```python
from build123d import *

# Parameters (mm, degrees)
SKETCH2_W                 = 80
SKETCH2_H                 = 211
SKETCH2_W_2               = 53.6
SKETCH2_H_2               = 11.7
BOSS_EXTRUDE1_DEPTH       = 2
M3X0_5_TAPPED_HOLE1_D     = 2.5
M3X0_5_TAPPED_HOLE1_DEPTH = 10
M3X0_5_TAPPED_HOLE1_TIP   = 0.751075774
SKETCH7_R                 = 3
CUT_EXTRUDE1_DEPTH        = 2


with BuildPart() as part:
    # Sketch2 → Boss-Extrude1 (new body)
    with BuildSketch(Plane.XY):
        with Locations((40, 105.5)):
            Rectangle(SKETCH2_W, SKETCH2_H)
        with Locations((40, 161.75)):
            Rectangle(SKETCH2_W_2, SKETCH2_H_2, mode=Mode.SUBTRACT)
    extrude(amount=BOSS_EXTRUDE1_DEPTH)

    # M3x0.5 Tapped Hole1
    with Locations(Plane(origin=(0, 0, 0), x_dir=(-1, 0, 0), z_dir=(0, 0, -1))):
        with Locations((-75, 196), (-5, 196), (-75, 23), (-5, 23)):
            Hole(M3X0_5_TAPPED_HOLE1_D / 2, depth=M3X0_5_TAPPED_HOLE1_DEPTH)
            with Locations((0, 0, -(M3X0_5_TAPPED_HOLE1_DEPTH + M3X0_5_TAPPED_HOLE1_TIP / 2))):  # 118° drill point
                Cone(0, M3X0_5_TAPPED_HOLE1_D / 2, M3X0_5_TAPPED_HOLE1_TIP, mode=Mode.SUBTRACT)

    # Sketch7 → Cut-Extrude1 (cut)
    with BuildSketch(Plane(origin=(0, 0, 0), x_dir=(-1, 0, 0), z_dir=(0, 0, -1))):
        with Locations((-75, 186)):
            Circle(SKETCH7_R)
        with Locations((-75, 139.2)):
            Circle(SKETCH7_R)
        with Locations((-75, 109.2)):
            Circle(SKETCH7_R)
        with Locations((-75, 79.2)):
            Circle(SKETCH7_R)
        with Locations((-75, 50.2)):
            Circle(SKETCH7_R)
        with Locations((-75, 30.2)):
            Circle(SKETCH7_R)
        with Locations((-5, 186)):
            Circle(SKETCH7_R)
        with Locations((-5, 139.2)):
            Circle(SKETCH7_R)
        with Locations((-5, 109.2)):
            Circle(SKETCH7_R)
        with Locations((-5, 79.2)):
            Circle(SKETCH7_R)
        with Locations((-5, 50.2)):
            Circle(SKETCH7_R)
        with Locations((-5, 30.2)):
            Circle(SKETCH7_R)
        with Locations((-70.3, 13)):
            Circle(SKETCH7_R)
        with Locations((-60, 205)):
            Circle(SKETCH7_R)
        with Locations((-20, 205)):
            Circle(SKETCH7_R)
        with Locations((-60, 6)):
            Circle(SKETCH7_R)
        with Locations((-20, 6)):
            Circle(SKETCH7_R)
        with Locations((-9.7, 13)):
            Circle(SKETCH7_R)
    extrude(amount=-CUT_EXTRUDE1_DEPTH, mode=Mode.SUBTRACT)


solid = part.part
```
The model under review builds one solid part; all positions refer to its coordinate system, in mm. Give positions to 0.01 mm unless a question says otherwise; leave off trailing zeros. Loops run counter-clockwise (first coordinate to the right, second up) from the corner with the lowest first, then second, coordinate; pieces in that order, holes last. Notation, with made-up numbers: (82.5, -12) - (101.5, -12) arc R25 cw to (101.5, 10) - close; hole circle Ø6 at (16.5, 87). An arc over 180 degrees is marked (long way). Answer as a JSON object with one key per item and string values.
Q1. To check wall thickness, follow line 1 along Y through (x, z) = (60, 0.9); line 2 along X through (y, z) = (205, 0.45); line 3 along Y through (x, z) = (50, 0.25). State the ranges of each line that lie inside material, in increasing order.
Worked out:
{"line 1": "y = 0 to 3, 9 to 155.9, 167.6 to 202, 208 to 211", "line 2": "x = 0 to 17, 23 to 57, 63 to 80", "line 3": "y = 0 to 155.9, 167.6 to 211"}
Q2. Add section B-B on z = 1. Count the separate pieces of the cut face and the enclosed holes in it, plus the area to 3 significant figures.
Worked out:
{"separate pieces": "1", "enclosed holes": "23", "area": "15,700 mm^2"}
Q3. Insertion check: pin 1 (8 mm diameter, centred on x = 75, y = 79.2, fed in from -Z). The pin has a flat end and moves straight along its axis. Give the tip position at first contact, or say it passes through.
Worked out:
{"pin 1": "stops at z = 0"}
Q4. Add section C-C on y = 30.2. State the section outline as (x, z) points.
Worked out:
{"outline": "(0, 0) - (2, 0) - (2, 2) - (0, 2) - close; (8, 0) - (72, 0) - (72, 2) - (8, 2) - close; (78, 0) - (80, 0) - (80, 2) - (78, 2) - close"}
Q5. Add section A-A on x = 20. State the section outline as (y, z) points.
Worked out:
{"outline": "(0, 0) - (3, 0) - (3, 2) - (0, 2) - close; (9, 0) - (155.9, 0) - (155.9, 2) - (9, 2) - close; (167.6, 0) - (202, 0) - (202, 2) - (167.6, 2) - close; (208, 0) - (211, 0) - (211, 2) - (208, 2) - close"}
Q6. Add section D-D on x = 46.5. State the section outline as (y, z) points.
Worked out:
{"outline": "(0, 0) - (155.9, 0) - (155.9, 2) - (0, 2) - close; (167.6, 0) - (211, 0) - (211, 2) - (167.6, 2) - close"}
Q7. Mouldability with a two-part tool opening along X and no side actions: class faces 1 (the cylindrical face through (20, 208, 1)), 2 (the flat face through (39, 107, 2)) as +X half, -X half, draft (parallel to the pull), parting line (faces both ways), or undercut.
Worked out:
{"face 1": "undercut", "face 2": "draft"}
